from build123d import *

# Parameters (mm, degrees)
SKETCH1_W           = 30
SKETCH1_H           = 38
BOSS_EXTRUDE1_DEPTH = 0.8
SKETCH2_R           = 1.109088316
SKETCH2_R_2         = 0.767029383
SKETCH2_R_3         = 0.775376329
SKETCH2_R_4         = 0.965264576
CUT_EXTRUDE1_DEPTH  = 0.8
SKETCH3_R           = 0.762390383
SKETCH3_W           = 4.894784697
SKETCH3_H           = 2.593636899
SKETCH3_W_2         = 4.192792091
SKETCH3_H_2         = 6.804733529
SKETCH3_W_3         = 3.597522217
SKETCH3_H_3         = 2.857060704
SKETCH3_W_4         = 3.52833422
SKETCH3_H_4         = 7.990285999
SKETCH3_W_5         = 4.960404455
SKETCH3_H_5         = 2.392024826
SKETCH3_W_6         = 2.649975693
SKETCH3_H_6         = 1.766675078
SKETCH3_W_7         = 2.778355341
SKETCH3_H_7         = 1.719515045
SKETCH3_W_8         = 1.492224114
SKETCH3_H_8         = 4.092690132
SKETCH3_W_9         = 2.214520185
SKETCH3_H_9         = 1.440440718
SKETCH3_W_10        = 2.082297707
SKETCH3_H_10        = 1.343633444
SKETCH3_W_11        = 2.964936673
SKETCH3_H_11        = 1.954523976
SKETCH3_W_12        = 3.040001034
SKETCH3_H_12        = 2.031411973
SKETCH3_W_13        = 3.147081738
SKETCH3_H_13        = 1.964784153
SKETCH3_W_14        = 3.191518467
SKETCH3_H_14        = 1.818199508
SKETCH3_W_15        = 1.580834587
SKETCH3_H_15        = 1.033148902
SKETCH3_W_16        = 1.585712642
SKETCH3_H_16        = 0.978957998
SKETCH3_W_17        = 1.469355228
SKETCH3_H_17        = 1.07248279
SKETCH3_W_18        = 1.436511349
SKETCH3_H_18        = 1.181213981
SKETCH3_W_19        = 1.43651135
SKETCH3_H_19        = 1.521795272
SKETCH3_W_20        = 9.81533928
SKETCH3_H_20        = 11.052195098
BOSS_EXTRUDE2_DEPTH = 0.8
SKETCH4_W           = 1.825068619
SKETCH4_H           = 1.589839684
SKETCH4_W_2         = 1.975600159
SKETCH4_W_3         = 1.455054018
SKETCH4_H_2         = 1.55750712
SKETCH4_W_4         = 1.850712573
SKETCH4_H_3         = 1.49055505
SKETCH4_W_5         = 1.966905423
SKETCH4_H_4         = 1.798635407
SKETCH4_W_6         = 1.927265264
SKETCH4_H_5         = 2.401166398
SKETCH4_W_7         = 2.040835962
SKETCH4_H_6         = 3.123215429
SKETCH4_W_8         = 2.990312219
SKETCH4_H_7         = 2.85468568
BOSS_EXTRUDE3_DEPTH = 0.8
SKETCH5_R           = 1.166233651
BOSS_EXTRUDE4_DEPTH = 2


with BuildPart() as part:
    # Sketch1 → Boss-Extrude1 (new body)
    with BuildSketch(Plane(origin=(0, 0, 0), x_dir=(1, 0, 0), z_dir=(0, 1, 0))):
        Rectangle(SKETCH1_W, SKETCH1_H)
    extrude(amount=BOSS_EXTRUDE1_DEPTH)

    # Sketch2 → Cut-Extrude1 (cut)
    with BuildSketch(Plane(origin=(0, 0.8, 0), x_dir=(1, 0, 0), z_dir=(0, 1, 0))):
        with Locations(Location((11.250748943, -15.842220292, 0), (0, 0, 270))):
            Circle(SKETCH2_R)
        with Locations(Location((-12.822379124, -15.842220292, 0), (0, 0, 270))):
            Circle(SKETCH2_R_2)
        with Locations(Location((12.359837258, 16.028797503, 0), (0, 0, 270))):
            Circle(SKETCH2_R_3)
        with Locations(Location((-12.822379124, 16.54551038, 0), (0, 0, 270))):
            Circle(SKETCH2_R_4)
    extrude(amount=-CUT_EXTRUDE1_DEPTH, mode=Mode.SUBTRACT)

    # Sketch3 → Boss-Extrude2 (add)
    with BuildSketch(Plane(origin=(0, 0.8, 0), x_dir=(1, 0, 0), z_dir=(0, 1, 0))):
        with Locations(Location((9.514606687, 14.257204648, 0), (0, 0, 270))):
            Circle(SKETCH3_R)
        with Locations((4.377365901, -11.445055136)):
            Rectangle(SKETCH3_W, SKETCH3_H)
        with Locations((-11.488143819, -7.293161754)):
            Rectangle(SKETCH3_W_2, SKETCH3_H_2)
        with Locations((4.377365901, -3.89079499)):
            Rectangle(SKETCH3_W_3, SKETCH3_H_3)
        with Locations((3.450098414, 3.595282667)):
            Rectangle(SKETCH3_W_4, SKETCH3_H_4)
        with Locations((4.921355444, 12.052974346)):
            Rectangle(SKETCH3_W_5, SKETCH3_H_5)
        with Locations((-6.265733234, -5.883849823)):
            Rectangle(SKETCH3_W_6, SKETCH3_H_6)
        with Locations((-6.230165426, -8.436309488)):
            Rectangle(SKETCH3_W_7, SKETCH3_H_7)
        with Locations((-0.464784197, -10.695528519)):
            Rectangle(SKETCH3_W_8, SKETCH3_H_8)
        with Locations((-6.296276665, -12.502715855)):
            Rectangle(SKETCH3_W_9, SKETCH3_H_9)
        with Locations((-6.230165426, -14.58062451)):
            Rectangle(SKETCH3_W_10, SKETCH3_H_10)
        with Locations((10.3743464, -11.611945846)):
            Rectangle(SKETCH3_W_11, SKETCH3_H_11)
        with Locations((10.351951393, -8.565924221)):
            Rectangle(SKETCH3_W_12, SKETCH3_H_12)
        with Locations((10.240052284, -5.711675816)):
            Rectangle(SKETCH3_W_13, SKETCH3_H_13)
        with Locations((10.066157491, -3.254157356)):
            Rectangle(SKETCH3_W_14, SKETCH3_H_14)
        with Locations((10.916850927, 1.828837055)):
            Rectangle(SKETCH3_W_15, SKETCH3_H_15)
        with Locations((10.739321253, 3.731847337)):
            Rectangle(SKETCH3_W_16, SKETCH3_H_16)
        with Locations((10.748827302, 5.668032924)):
            Rectangle(SKETCH3_W_17, SKETCH3_H_17)
        with Locations((10.56243198, 7.774708171)):
            Rectangle(SKETCH3_W_18, SKETCH3_H_18)
        with Locations((10.500800241, 10.042163174)):
            Rectangle(SKETCH3_W_19, SKETCH3_H_19)
        with Locations((-9.076372897, 6.688794027)):
            Rectangle(SKETCH3_W_20, SKETCH3_H_20)
    extrude(amount=BOSS_EXTRUDE2_DEPTH)

    # Sketch4 → Boss-Extrude3 (add)
    with BuildSketch(Plane(origin=(0, 0.8, 0), x_dir=(1, 0, 0), z_dir=(0, 1, 0))):
        with Locations((-2.768458169, -15.760115658)):
            Rectangle(SKETCH4_W, SKETCH4_H)
        with Locations((-0.202584614, -15.760115658)):
            Rectangle(SKETCH4_W_2, SKETCH4_H)
        with Locations((1.903702303, -15.77628194)):
            Rectangle(SKETCH4_W_3, SKETCH4_H_2)
        with Locations((4.144992677, -15.837154802)):
            Rectangle(SKETCH4_W_4, SKETCH4_H_3)
        with Locations((7.414099695, 1.774450018)):
            Rectangle(SKETCH4_W_5, SKETCH4_H_4)
        with Locations((7.283749146, 4.735498446)):
            Rectangle(SKETCH4_W_6, SKETCH4_H_5)
        with Locations((7.104971851, 8.134512532)):
            Rectangle(SKETCH4_W_7, SKETCH4_H_6)
        with Locations((-3.066161458, -3.210239912)):
            Rectangle(SKETCH4_W_8, SKETCH4_H_7)
    extrude(amount=BOSS_EXTRUDE3_DEPTH)

    # Sketch5 → Boss-Extrude4 (add)
    with BuildSketch(Plane(origin=(0, 0.8, 0), x_dir=(1, 0, 0), z_dir=(0, 1, 0))):
        with Locations(Location((-10.677990128, -14.091680692, 0), (0, 0, 270))):
            Circle(SKETCH5_R)
    extrude(amount=BOSS_EXTRUDE4_DEPTH)


solid = part.part
CAD build for the part. Positions are in the model's coordinates, mm. A direction names the side the tool comes from. Round coordinates to 2 decimals unless told otherwise and drop trailing zeros. Write each loop counter-clockwise with the first axis right and the second up, starting at its lowest first coordinate (ties: lowest second). Pieces come first, ordered by that corner, then holes. Notation, with made-up numbers: M -20,47 L 16,47 A31 ccw 16,84 Z; hole C -24.5,-38 d11. An arc over 180 degrees is marked long. Use a Markdown table: item, result. Add a question column.
1. Flat gauge pins, fed straight in: P1, Ø0.6, axis at y = 1.5, z = -8, coming from the +X side; P2, Ø0.9, axis at y = 1.5, z = 15.5, coming from the +X side; P3, Ø0.9, axis at x = 3.5, y = 1.5, coming from the +Z side; P4, Ø1, axis at x = 10.5, y = 1, coming from the -Z side. Where does each tip first touch, or does it go through?
2. 3-axis set-ups, long thin cutter, end or side, ignore diameter. For faces 4 (the face through (2, 1.6, 16)), 5 (the face through (-12, 1.6, 7)), 6 (the face through (11, 1.6, -2)): which of +Z, -Z, +X, -X, +Y, -Y reach the whole face in a straight line?
3. Slice it at B-B on y = 2.2. Give the cut face in (x, z).
4. Drill centre lines: probe 1 along Z at (x, y) = (-6.25, 1.5); probe 2 along Z at (x, y) = (9.5, 0.9); probe 3 along Z at (x, y) = (-0.5, 1.1). Where is each one in solid material? Low to high.
5. Slice it at A-A on z = 3. Give the cut face in (x, y), then the cut area to 3 significant figures.
6. Pull direction X, two halves, no side cores. Call faces 1 (the face through (-13.289, 0.406, 15.234)), 2 (the face through (-12.78, 0.41, -17.51)), 3 (the face through (-3, 1.6, 3)): released by +X, released by -X, zero draft, split by the parting line, or undercut.
Reply:
| question | item | result |
|---|---|---|
| 1 | P1 | stops at x = 11.28 |
| 1 | P2 | stops at x = 5.07 |
| 1 | P3 | stops at z = 16.58 |
| 1 | P4 | stops at z = -19 |
| 2 | face 4 | +Z, -Z, +X, +Y |
| 2 | face 5 | -Z, +X, -X, +Y |
| 2 | face 6 | +Z, -Z, +X, -X, +Y |
| 3 | outline | C -10.68,14.09 d2.33 |
| 4 | probe 1 | z = -12.21 to -1.16, 5 to 6.77, 7.58 to 9.3, 11.78 to 13.22, 13.91 to 15.25 |
| 4 | probe 2 | z = -15.02 to -13.49, 2.35 to 4.16, 4.73 to 6.69, 7.55 to 9.58, 10.63 to 12.59 |
| 4 | probe 3 | z = 8.65 to 12.74, 14.97 to 16.56 |
| 5 | outline | M -15,0 L 15,0 L 15,0.8 L 11.66,0.8 L 11.66,1.6 L 8.47,1.6 L 8.47,0.8 L 6.18,0.8 L 6.18,1.6 L 2.58,1.6 L 2.58,0.8 L -1.57,0.8 L -1.57,1.6 L -4.56,1.6 L -4.56,0.8 L -15,0.8 Z |
| 5 | area | 31.8 mm^2 |
| 6 | face 1 | undercut |
| 6 | face 2 | undercut |
| 6 | face 3 | zero draft |
